```python
from build123d import *

# Parameters (mm, degrees)
ESBO_O1_R                = 25
RESSALTO_EXTRUS_O1_DEPTH = 12.5
ESBO_O3_R                = 11.5
CORTE_EXTRUS_O1_DEPTH    = 25
ESBO_O4_R                = 17.5
CORTE_EXTRUS_O2_DEPTH    = 18
CHANFRO1_SIZE            = 0.5
ESBO_O5_W                = 1.6
ESBO_O5_H                = 18.5


with BuildPart() as part:
    # Esboço1 → Ressalto-extrusão1 (new, symmetric)
    with BuildSketch(Plane.XY):
        Circle(ESBO_O1_R)
    extrude(amount=RESSALTO_EXTRUS_O1_DEPTH, both=True)

    # Esboço3 → Corte-extrusão1 (cut)
    with BuildSketch(Plane.XY.offset(12.5)):
        Circle(ESBO_O3_R)
    extrude(amount=-CORTE_EXTRUS_O1_DEPTH, mode=Mode.SUBTRACT)

    # Esboço4 → Corte-extrusão2 (cut)
    with BuildSketch(Plane.XY.offset(12.5)):
        Circle(ESBO_O4_R)
    extrude(amount=-CORTE_EXTRUS_O2_DEPTH, mode=Mode.SUBTRACT)

    # Chanfro1
    chanfro1_edges = [part.edges().sort_by_distance(p)[0] for p in [
        (-17.5, 0, 12.5),
        (-11.5, 0, -5.5),
        (-25, 0, -12.5),
        (-25, 0, 12.5),
        (-11.5, 0, -12.5),
    ]]
    chamfer(chanfro1_edges, length=CHANFRO1_SIZE)

    # Esboço5 → Corte-Revolução2 (revolve, cut)
    with BuildSketch(Plane(origin=(0, 0, 0), x_dir=(0, 0, -1), z_dir=(1, 0, 0)), mode=Mode.PRIVATE) as corte_revolu_o2_sk:
        with Locations((-6.3, 9.25)):
            Rectangle(ESBO_O5_W, ESBO_O5_H)
    revolve(corte_revolu_o2_sk.sketch.rotate(Axis((0, 0, 5.5), (0, 0, 1)), 270), axis=Axis((0, 0, 5.5), (0, 0, 1)), mode=Mode.SUBTRACT)


solid = part.part
```
Geometry: final body of the model. Coordinates: model frame, mm. A direction names the side the tool comes from. Coordinates: 2 decimals unless noted, no trailing zeros. Order: outer loops, then holes, each group sorted by start corner. A loop starts at its lowest first (then second) coordinate and runs counter-clockwise, first axis right, second up. Notation, with made-up numbers: (82, 5) -> (111, 5) arc R21 ccw to (111, 43) -> close; hole circle Ø1 at (-14.75, 9.5). An arc over 180 degrees is marked (long way). Write item = value, one per line.
(1) Pull-direction query (Z, two-part tool) for faces 4 (the flat face through (11, -14, 7.1)), 5 (the flat face through (11, 6, -12.5)), 6 (the flat face through (-12, -4, -5.5)); classes: pulls with the +Z half, pulls with the -Z half, needs draft (parallel to the pull), parting line crosses it, or undercut.
Solved:
face_4 = undercut
face_5 = pulls with the -Z half
face_6 = pulls with the +Z half
(2) Pin query (flat end, axial travel): pin 1 Ø3 at (x, y) = (-9.5, -5) entering from +Z; pin 2 Ø1.5 at (y, z) = (8, -8) entering from +X; pin 3 Ø1.5 at (x, z) = (-18, -4) entering from -Y; pin 4 Ø11 at (x, y) = (-7, -5.5) entering from -Z. Return the tip coordinate at first contact, or that it passes through.
Solved:
pin_1 = -5.5
pin_2 = 23.93
pin_3 = -18.1
pin_4 = -12.5
(3) Access query for faces 1 (the cylindrical face through (-1.5, 11.4, -9)), 2 (the cylindrical face through (-13.887, -10.648, 0.077)), 3 (the cylindrical face through (17.089, -7.086, 6.289)). Directions: +Z, -Z, +X, -X, +Y, -Y. A direction counts if a zero-diameter tool reaches every point of the face in a straight line with its end or side. Return the directions, or none.
Solved:
face_1 = +Z, -Z
face_2 = +Z
face_3 = none
(4) Line query: line 1 (Y direction, x = 0, z = -9.85); line 2 (Y direction, x = 0, z = 1.5); line 3 (Z direction, x = 7.5, y = 10.5). Output: solid intervals per line, ascending.
Solved:
line_1 = -25 to -11.5, 11.5 to 25
line_2 = -25 to -17.5, 17.5 to 25
line_3 = -12.5 to -5.5
(5) Cut plane C-C on z = -3.25. Return loops of the section in (x, y), plus the area to 3 significant figures.
Solved:
outline = circle Ø50 at (0, 0); hole circle Ø35 at (0, 0)
area = 1,000 mm²
